Geometry check sheet. Reference: the model listing, model coordinates, mm. Face numbers are marked on the shaded views. A direction names the side the tool comes from. Coordinates: 2 decimals unless noted, no trailing zeros. Write each loop counter-clockwise with the first axis right and the second up, starting at its lowest first coordinate (ties: lowest second). Pieces come first, ordered by that corner, then holes. Notation, with made-up numbers: (67.25, 11.5) -> (76.25, 11.5) arc R22 cw to (76.25, 45.5) -> close; hole circle Ø2 at (45.25, 7.25). An arc over 180 degrees is marked (long way). One line per question, with ' | ' between items.
from build123d import *

# Parameters (mm, degrees)
BOSS_EXTRUDE1_DEPTH            = 8.75
M3_CLEARANCE_HOLE1_D           = 2
CUT_EXTRUDE2_REACH             = 66.481
SKETCH5_W                      = 1.25
SKETCH5_H                      = 5
SKETCH7_W                      = 15.88
SKETCH7_H                      = 3
CUT_EXTRUDE4_DEPTH             = 50
CBORE_FOR_M3_SHCS1_D           = 3.4
CBORE_FOR_M3_SHCS1_CBORE_D     = 6.5
CBORE_FOR_M3_SHCS1_CBORE_DEPTH = 3
FILLET1_R                      = 1
SKETCH12_R                     = 7.5
CUT_EXTRUDE5_DEPTH             = 5.75
CBORE_FOR_M3_SHCS2_D           = 3.4
CBORE_FOR_M3_SHCS2_CBORE_D     = 6.5
CBORE_FOR_M3_SHCS2_CBORE_DEPTH = 53


with BuildPart() as part:
    # Sketch1 → Boss-Extrude1 (new body)
    with BuildSketch(Plane.XY):
        Polygon((0, 0), (32.5, 0), (32.5, 4.239766082), (32.5, 55), (16.62, 55), (16.62, 5), (0, 5), align=None)
    extrude(amount=BOSS_EXTRUDE1_DEPTH)

    # M3 Clearance Hole1 (through all)
    with Locations(Plane.XY.offset(8.75)):
        with Locations((29.68, 52.275), (19.52, 30)):
            Hole(M3_CLEARANCE_HOLE1_D / 2)

    # Cut-Extrude2: up to this face of the body (flat: up to its plane)
    cut_extrude2_end = Plane(part.part.faces().sort_by_distance((32.5, 27.5, 4.375))[0])
    # Sketch5 → Cut-Extrude2 (cut, up to the picked face)
    with BuildSketch(Plane.ZY, mode=Mode.PRIVATE) as cut_extrude2_sk1:
        with Locations((8.125, 2.5)):
            Rectangle(SKETCH5_W, SKETCH5_H)
    cut_extrude2_tool1 = split(extrude(cut_extrude2_sk1.sketch, amount=-CUT_EXTRUDE2_REACH, mode=Mode.PRIVATE), bisect_by=cut_extrude2_end, keep=Keep.BOTH, mode=Mode.PRIVATE)
    add(cut_extrude2_tool1.solids().sort_by(Axis((0, 2.5, 8.125), (1, 0, 0)))[0], mode=Mode.SUBTRACT)

    # Sketch7 → Cut-Extrude4 (cut)
    with BuildSketch(Plane(origin=(0, 55, 0), x_dir=(1, 0, 0), z_dir=(0, 1, 0))):
        with Locations((24.56, -1.5)):
            Rectangle(SKETCH7_W, SKETCH7_H)
    extrude(amount=-CUT_EXTRUDE4_DEPTH, mode=Mode.SUBTRACT)

    # CBORE for M3 SHCS1 (through all)
    with Locations(Plane(origin=(0, 5, 0), x_dir=(1, 0, 0), z_dir=(0, 1, 0))):
        with Locations((4.2, -3.75)):
            CounterBoreHole(CBORE_FOR_M3_SHCS1_D / 2, CBORE_FOR_M3_SHCS1_CBORE_D / 2, CBORE_FOR_M3_SHCS1_CBORE_DEPTH)

    # Fillet1
    fillet1_edges = [part.edges().sort_by_distance(p)[0] for p in [
        (16.62, 55, 5.875),
        (32.5, 55, 5.875),
        (16.62, 5, 5.25),
        (0, 2.5, 7.5),
        (32.5, 2.5, 7.5),
        (24.56, 5, 3),
        (32.5, 2.5, 0),
        (0, 2.5, 0),
    ]]
    fillet(fillet1_edges, radius=FILLET1_R)

    # Sketch12 → Cut-Extrude5 (cut)
    with BuildSketch(Plane.XY.offset(8.75)):
        with Locations((12.7, 12.7)):
            Circle(SKETCH12_R)
    extrude(amount=-CUT_EXTRUDE5_DEPTH, mode=Mode.SUBTRACT)

    # CBORE for M3 SHCS2 (through all)
    with Locations(Plane(origin=(0, 55, 0), x_dir=(1, 0, 0), z_dir=(0, 1, 0))):
        with Locations((24.2, -3.75)):
            CounterBoreHole(CBORE_FOR_M3_SHCS2_D / 2, CBORE_FOR_M3_SHCS2_CBORE_D / 2, CBORE_FOR_M3_SHCS2_CBORE_DEPTH)


solid = part.part
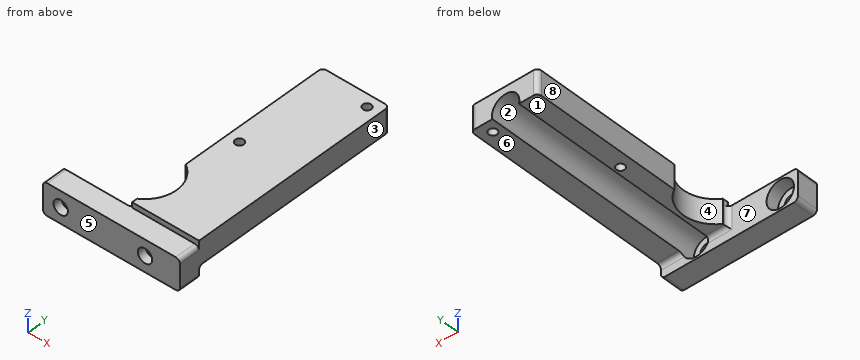
1. Material ranges on line 1 (Z direction, x = 4.2, y = 2.6); line 2 (Z direction, x = 4.2, y = 0.95); line 3 (Y direction, x = 19.52, z = 6.3), recorded low to high. Write a range as from..to.
Worked answers:
line 1: 0..0.5, 7..7.5 | line 2: 0..2.05, 5.45..7.5 | line 3: 0..9.58, 15.82..29, 31..55
2. Go/stop test with flat-tipped pins: P1, Ø5, axis at y = 35, z = 1.5, coming from the -X side; P2, Ø2.5, axis at x = 31, y = 40, coming from the -Z side; P3, Ø1.6, axis at x = 19.52, y = 30, coming from the +Z side; P4, Ø3, axis at x = 4.5, z = 8, coming from the +Y side. Record where each tip stops, or that it passes through.
Worked answers:
P1: x = 16.62 | P2: z = 3 | P3: through | P4: y = 5
3. Cross-section at A-A on x = 4.2. Record the boundary of the cut face in (y, z).
Worked answers:
outline: (0, 0) -> (5, 0) -> (5, 0.5) -> (2, 0.5) -> (2, 2.05) -> (0, 2.05) -> close; (0, 5.45) -> (2, 5.45) -> (2, 7) -> (5, 7) -> (5, 7.5) -> (0, 7.5) -> close
4. Mould release check, pull along X, two halves, no side actions. Record for the marked faces 1, 2, 3 and 4: released by +X, released by -X, zero draft, split by the parting line, or undercut.
Worked answers:
face 1: zero draft | face 2: undercut | face 3: released by +X | face 4: released by -X
5. Cross-section at C-C on y = 24. Record the boundary of the cut face in (x, z), and give its area (3 significant figures).
Worked answers:
outline: (16.62, 3) -> (21.04, 3) arc R3.25 cw (long way) to (27.36, 3) -> (32.5, 3) -> (32.5, 8.75) -> (16.62, 8.75) -> close | area: 69.9 mm²
6. Cross-section at D-D on x = 24.2. Record the boundary of the cut face in (y, z).
Worked answers:
outline: (0, 0) -> (5, 0) -> (5, 0.5) -> (2, 0.5) -> (2, 2.05) -> (0, 2.05) -> close; (0, 5.45) -> (2, 5.45) -> (2, 7) -> (55, 7) -> (55, 8.75) -> (5, 8.75) -> (5, 7.5) -> (0, 7.5) -> close
7. Tool access check on the marked faces 5, 6, 7 and 8. Record the directions out of +Z, -Z, +X, -X, +Y, -Y that give a thin tool (end or side, any length) a straight path to the whole face; none if there is none.
Worked answers:
face 5: +Z, -Z, +X, -X, -Y | face 6: -Z, +X, -X, +Y | face 7: -Z, -X, +Y | face 8: +Z, -Z, -X, +Y
8. Cross-section at B-B on z = 3.75. Give the number of separate pieces and of enclosed holes in the cut face, and give its area (3 significant figures).
Worked answers:
separate pieces: 3 | enclosed holes: 2 | area: 540 mm²
